CAD build for the part. Positions are in the model's coordinates, mm. A direction names the side the tool comes from. Give positions to 0.01 mm unless a question says otherwise; leave off trailing zeros. Order: outer loops, then holes, each group sorted by start corner. A loop starts at its lowest first (then second) coordinate and runs counter-clockwise, first axis right, second up.
Item 1: Band-saw the part on A-A on z = 1. Give the cut face in (x, y).
Item 2: Band-saw the part on B-B on y = 2.35. Give the cut face in (x, z), plus the area to 3 significant figures.
Item 3: Flat gauge pins, fed straight in: P1, Ø0.9, axis at x = 5.5, y = 1, coming from the +Z side; P2, Ø0.9, axis at y = 2, z = 1, coming from the +X side; P3, Ø2.5, axis at x = 10, z = -13, coming from the +Y side. Where does each tip first touch, or does it go through?
Item 4: Band-saw the part on C-C on x = 10. Give the cut face in (y, z), plus the area to 3 significant figures.
Item 5: Band-saw the part on D-D on z = -13.5. Give the cut face in (x, y).
Item 6: Two-plate mould, pull along Z, no slides. Class faces 1 (the flat face through (35, 1, -20)), 2 (the flat face through (0, 1, -10)), 3 (the flat face through (35, 1, 0)), 4 (the flat face through (20, 1, -5)): released by +Z, released by -Z, zero draft, split by the parting line, or undercut.
Item 7: Which spindle directions (+Z, -Z, +X, -X, +Y, -Y) get a long thin tool onto all of the face, cutting with end or side? Do faces 5 (the flat face through (35, 0, -9)), 6 (the flat face through (51.5, 1, -10)), 7 (the flat face through (50, 1, 2)), 8 (the flat face through (27.5, 1, 2)), 9 (the flat face through (10, 1, 0)). Say none if no direction does.
Item 8: Wall check: L1, parallel to X at y = 0.95, z = -13; L2, parallel to X at y = 2.5, z = -7; L3, parallel to Z at x = 60, y = 1.3. Give the ranges that are in metal, low to high.
```python
from build123d import *

# Parameters (mm, degrees)
SKETCH1_R           = 2
SKETCH1_W           = 3
SKETCH1_H           = 10
BOSS_EXTRUDE1_DEPTH = 3


with BuildPart() as part:
    # Sketch1 → Boss-Extrude1 (new body)
    with BuildSketch(Plane(origin=(0, 0, 0), x_dir=(1, 0, 0), z_dir=(0, 1, 0))):
        Polygon((0, 0), (20, 0), (20, -3), (27.5, -3), (27.5, 0), (42.5, 0), (42.5, -3), (50, -3), (50, 0), (70, 0), (70, 20), (0, 20), align=None)
        with Locations(Location((10, 13, 0), (0, 0, 270))):
            Circle(SKETCH1_R, mode=Mode.SUBTRACT)
        with Locations(Location((60, 13, 0), (0, 0, 90))):
            Circle(SKETCH1_R, mode=Mode.SUBTRACT)
        with Locations((20, 10)):
            Rectangle(SKETCH1_W, SKETCH1_H, mode=Mode.SUBTRACT)
        with Locations((50, 10)):
            Rectangle(SKETCH1_W, SKETCH1_H, mode=Mode.SUBTRACT)
    extrude(amount=BOSS_EXTRUDE1_DEPTH)


solid = part.part
```
The answers:
1. outline: (20, 0) - (27.5, 0) - (27.5, 3) - (20, 3) - close; (42.5, 0) - (50, 0) - (50, 3) - (42.5, 3) - close
2. outline: (0, -20) - (70, -20) - (70, 0) - (50, 0) - (50, 3) - (42.5, 3) - (42.5, 0) - (27.5, 0) - (27.5, 3) - (20, 3) - (20, 0) - (0, 0) - close; hole circle Ø4 at (10, -13); hole (18.5, -15) - (21.5, -15) - (21.5, -5) - (18.5, -5) - close; hole (48.5, -15) - (51.5, -15) - (51.5, -5) - (48.5, -5) - close; hole circle Ø4 at (60, -13)
2. area: 1,360 mm2
3. P1: stops at z = 0
3. P2: stops at x = 50
3. P3: passes through
4. outline: (0, -20) - (3, -20) - (3, -15) - (0, -15) - close; (0, -11) - (3, -11) - (3, 0) - (0, 0) - close
4. area: 48.0 mm2
5. outline: (0, 0) - (8.06, 0) - (8.06, 3) - (0, 3) - close; (11.94, 0) - (18.5, 0) - (18.5, 3) - (11.94, 3) - close; (21.5, 0) - (48.5, 0) - (48.5, 3) - (21.5, 3) - close; (51.5, 0) - (58.06, 0) - (58.06, 3) - (51.5, 3) - close; (61.94, 0) - (70, 0) - (70, 3) - (61.94, 3) - close
6. face 1: released by -Z
6. face 2: zero draft
6. face 3: released by +Z
6. face 4: undercut
7. face 5: +Z, -Z, +X, -X, -Y
7. face 6: +Y, -Y
7. face 7: +Z, +X, +Y, -Y
7. face 8: +Z, +Y, -Y
7. face 9: +Z, -X, +Y, -Y
8. L1: x = 0 to 8, 12 to 18.5, 21.5 to 48.5, 51.5 to 58, 62 to 70
8. L2: x = 0 to 18.5, 21.5 to 48.5, 51.5 to 70
8. L3: z = -20 to -15, -11 to 0
